CAD build for the part. Positions are in the model's coordinates, mm. Round coordinates to 2 decimals unless told otherwise and drop trailing zeros. Loops run counter-clockwise (first coordinate to the right, second up) from the corner with the lowest first, then second, coordinate; pieces in that order, holes last. Notation, with made-up numbers: M 67.25,-14 L 84.25,-14 A4 cw 84.25,-9 Z; hole C 30.25,18 d11. An arc over 180 degrees is marked long. Use a Markdown table: item, result. Add a question column.
(1) Band-saw the part on C-C, the plane z = 1482.5. Write the cut outline in (x, y) (3 decimals).
(2) Band-saw the part on B-B, the plane x = 12.5. Write the cut outline in (y, z) (3 decimals), and give its area (3 significant figures).
(3) Band-saw the part on A-A, the plane y = 27. Write the cut outline in (x, z) (3 decimals).
(4) Wall check: L1, parallel to Y at x = -22, z = 1785 (3 decimals); L2, parallel to Y at x = -58, z = 1455. Give the ranges that are in metal, low to high.
from build123d import *

# Parameters (mm, degrees)
F1_DEPTH      = 2413
F3_DEPTH      = 76.201
F3_DEPTH_BACK = 76.201


with BuildPart() as f1:
    # F0 (on Top) → F1 (new body)
    with BuildSketch(Plane.XY):
        with BuildLine():
            ThreePointArc((-76.2, -57.15), (-70.6203841816, -70.6203841816), (-57.15, -76.2))
            Line((-57.15, -76.2), (57.15, -76.2))
            ThreePointArc((57.15, -76.2), (70.6203841816, -70.6203841816), (76.2, -57.15))
            Line((76.2, -57.15), (76.2, 57.15))
            ThreePointArc((76.2, 57.15), (70.6203841816, 70.6203841816), (57.15, 76.2))
            Line((57.15, 76.2), (-57.15, 76.2))
            ThreePointArc((-57.15, 76.2), (-70.6203841816, 70.6203841816), (-76.2, 57.15))
            Line((-76.2, 57.15), (-76.2, -57.15))
        make_face()
        with BuildLine():
            Line((57.15, -66.675), (-57.15, -66.675))
            ThreePointArc((-57.15, -66.675), (-63.8851920908, -63.8851920908), (-66.675, -57.15))
            Line((-66.675, -57.15), (-66.675, 57.15))
            ThreePointArc((-66.675, 57.15), (-63.8851920908, 63.8851920908), (-57.15, 66.675))
            Line((-57.15, 66.675), (57.15, 66.675))
            ThreePointArc((57.15, 66.675), (63.8851920908, 63.8851920908), (66.675, 57.15))
            Line((66.675, 57.15), (66.675, -57.15))
            ThreePointArc((66.675, -57.15), (63.8851920908, -63.8851920908), (57.15, -66.675))
        make_face(mode=Mode.SUBTRACT)
    extrude(amount=F1_DEPTH)

    # F2 (on Right) → F3 (cut, two sides)
    with BuildSketch(Plane.YZ) as f3_sk:
        Polygon((76.2, 2413), (-76.2, 2413), (-76.2, 2260.6), align=None)
    extrude(amount=-F3_DEPTH, mode=Mode.SUBTRACT)
    extrude(f3_sk.sketch, amount=F3_DEPTH_BACK, mode=Mode.SUBTRACT)


solid = f1.part
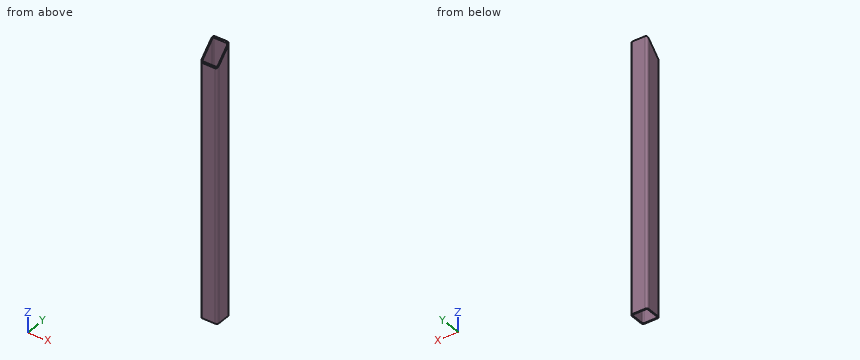
Return value:
| question | item | result |
|---|---|---|
| 1 | outline | M -76.2,-57.15 A19.05 ccw -57.15,-76.2 L 57.15,-76.2 A19.05 ccw 76.2,-57.15 L 76.2,57.15 A19.05 ccw 57.15,76.2 L -57.15,76.2 A19.05 ccw -76.2,57.15 Z; hole M -66.675,-57.15 A9.525 ccw -57.15,-66.675 L 57.15,-66.675 A9.525 ccw 66.675,-57.15 L 66.675,57.15 A9.525 ccw 57.15,66.675 L -57.15,66.675 A9.525 ccw -66.675,57.15 Z |
| 2 | outline | M -76.2,0 L -66.675,0 L -66.675,2270.125 L -76.2,2260.6 Z; M 66.675,0 L 76.2,0 L 76.2,2413 L 66.675,2403.475 Z |
| 2 | area | 44,500 mm^2 |
| 3 | outline | M -76.2,0 L -66.675,0 L -66.675,2363.8 L -76.2,2363.8 Z; M 66.675,0 L 76.2,0 L 76.2,2363.8 L 66.675,2363.8 Z |
| 4 | L1 | -76.2 to -66.675, 66.675 to 76.2 |
| 4 | L2 | -76.18 to -66.64, 66.64 to 76.18 |
